Study the drawing (mm; zero at the part's minimum x, y, z) and answer. A direction names the side the tool comes from. Give positions to 0.01 mm unless a question says otherwise; leave off trailing zeros. Write each loop counter-clockwise with the first axis right and the second up, starting at its lowest first coordinate (ties: lowest second). Pieces come first, ordered by that corner, then holes. Notation, with made-up numbers: (11.25, -14.75) -> (60.25, -14.75) arc R20 ccw to (60.25, -5.75) -> close; hole circle Ø1 at (73, 48). An arc over 180 degrees is marked (long way). Put each result on its own line as item: value. Start each with the question number.
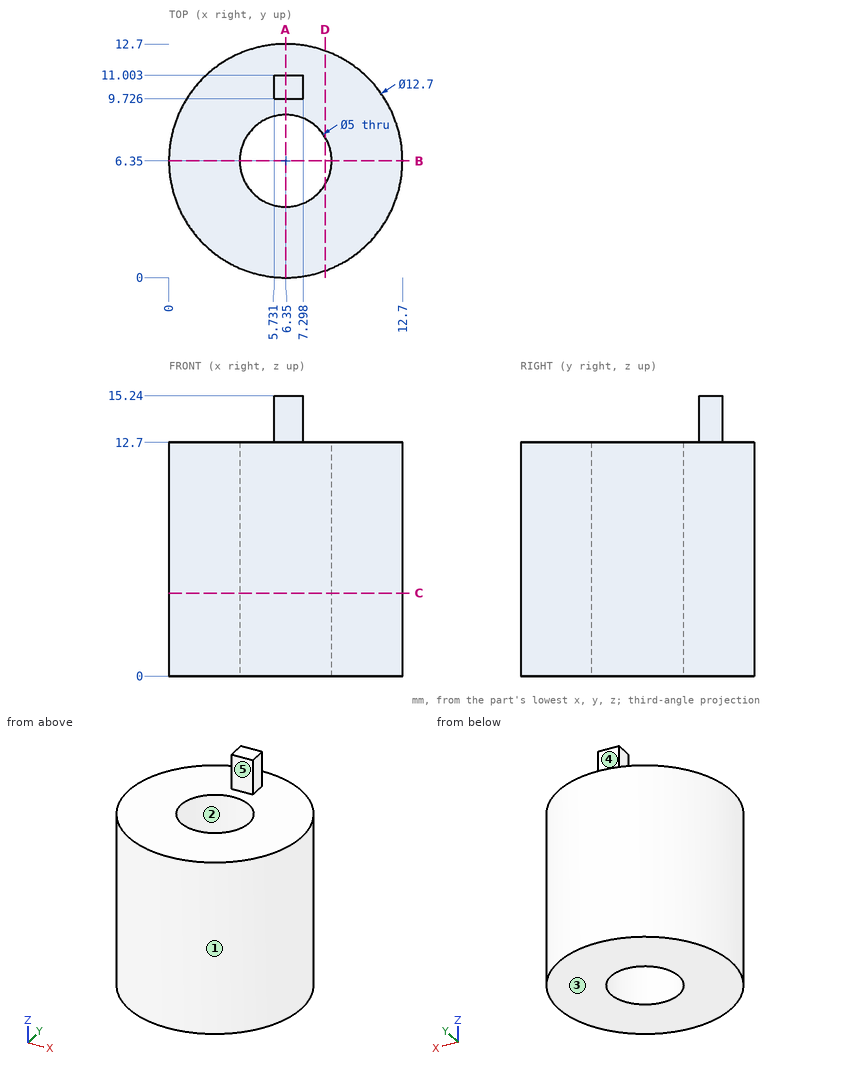
1) For the marked faces 4 and 5, determine the directions among +Z, -Z, +X, -X, +Y, -Y from which every point of the face is accessible in a straight line to the end or side of a thin tool.
2) A cutting plane is placed at C-C on z = 4.5. Give the vertices of the cut face in (x, y).
3) A cutting plane is placed at A-A on x = 6.35. Give the vertices of the cut face in (y, z), and give its area (3 significant figures).
4) Straight lines are drawn through the part: line 1 (Y direction, x = 6.35, z = 5.75); line 2 (Z direction, x = 10.5, y = 4.75); line 3 (X direction, y = 4.5, z = 9) (1 decimal). For each, find the intervals that lie inside material, in ascending order. Write a range as [from, to].
5) Each of these flat-tipped pins is pushed along its axis until it touches: pin 1 Ø1.3 at (x, z) = (6.5, 14) entering from +Y; pin 2 Ø1 at (x, z) = (9.5, 12.5) entering from -Y; pin 3 Ø0.8 at (x, z) = (6, 14) entering from -Y. Where does it stop, or does it pass through?
6) A cutting plane is placed at D-D on x = 8.5. Give the vertices of the cut face in (y, z) (1 decimal).
7) For a pull along Y with two mould halves and no side action, classify the marked faces 1, 2 and 3 as pulls with the +Y half, pulls with the -Y half, needs draft (parallel to the pull), parting line crosses it, or undercut.
8) A cutting plane is placed at B-B on y = 6.35. Give the vertices of the cut face in (x, z).
Results found:
1. face 4: +Z, +X, -X, +Y
1. face 5: +Z, +X, -X, -Y
2. outline: circle Ø12.7 at (6.35, 6.35); hole circle Ø5 at (6.35, 6.35)
3. outline: (0, 0) -> (3.85, 0) -> (3.85, 12.7) -> (0, 12.7) -> close; (8.85, 0) -> (12.7, 0) -> (12.7, 12.7) -> (11, 12.7) -> (11, 15.24) -> (9.73, 15.24) -> (9.73, 12.7) -> (8.85, 12.7) -> close
3. area: 101 mm²
4. line 1: y = [0, 3.85], [8.85, 12.7]
4. line 2: z = [0, 12.7]
4. line 3: x = [0.3, 4.7], [8, 12.4]
5. pin 1: stops at y = 11
5. pin 2: stops at y = 0.58
5. pin 3: stops at y = 9.73
6. outline: (0.4, 0) -> (5.1, 0) -> (5.1, 12.7) -> (0.4, 12.7) -> close; (7.6, 0) -> (12.3, 0) -> (12.3, 12.7) -> (7.6, 12.7) -> close
7. face 1: parting line crosses it
7. face 2: undercut
7. face 3: needs draft
8. outline: (0, 0) -> (3.85, 0) -> (3.85, 12.7) -> (0, 12.7) -> close; (8.85, 0) -> (12.7, 0) -> (12.7, 12.7) -> (8.85, 12.7) -> close
